```python
from build123d import *

# Parameters (mm, degrees)
SKETCH1_R                               = 159
SKETCH1_R_2                             = 121
BOSS_EXTRUDE1_DEPTH                     = 10
CBORE_FOR_M5_HEX_HEAD_BOLT2_D           = 6
CBORE_FOR_M5_HEX_HEAD_BOLT2_DEPTH       = 13
CBORE_FOR_M5_HEX_HEAD_BOLT2_CBORE_D     = 12
CBORE_FOR_M5_HEX_HEAD_BOLT2_CBORE_DEPTH = 6
CBORE_FOR_M5_HEX_HEAD_BOLT2_TIP         = 1.802581857


with BuildPart() as part:
    # Sketch1 → Boss-Extrude1 (new body)
    with BuildSketch(Plane(origin=(0, 0, 0), x_dir=(0, 0, -1), z_dir=(1, 0, 0))):
        Circle(SKETCH1_R)
        Circle(SKETCH1_R_2, mode=Mode.SUBTRACT)
    extrude(amount=BOSS_EXTRUDE1_DEPTH)

    # CBORE for M5 Hex Head Bolt2
    with Locations(Plane.ZY):
        with Locations((0, 150), (129.903810568, 75), (129.903810568, -75), (0, -150), (-129.903810568, -75), (-129.903810568, 75), (0, 0)):
            CounterBoreHole(CBORE_FOR_M5_HEX_HEAD_BOLT2_D / 2, CBORE_FOR_M5_HEX_HEAD_BOLT2_CBORE_D / 2, CBORE_FOR_M5_HEX_HEAD_BOLT2_CBORE_DEPTH, depth=CBORE_FOR_M5_HEX_HEAD_BOLT2_DEPTH)
            with Locations((0, 0, -(CBORE_FOR_M5_HEX_HEAD_BOLT2_DEPTH + CBORE_FOR_M5_HEX_HEAD_BOLT2_TIP / 2))):  # 118° drill point
                Cone(0, CBORE_FOR_M5_HEX_HEAD_BOLT2_D / 2, CBORE_FOR_M5_HEX_HEAD_BOLT2_TIP, mode=Mode.SUBTRACT)


solid = part.part
```
Design review of the part built by this model. Coordinates are the model's own, in mm. A direction names the side the tool comes from. Give positions to 0.01 mm unless a question says otherwise; leave off trailing zeros. Loops run counter-clockwise (first coordinate to the right, second up) from the corner with the lowest first, then second, coordinate; pieces in that order, holes last. Notation, with made-up numbers: (55.25, -21) -> (112.25, -21) arc R28 cw to (112.25, 2) -> close; hole circle Ø11 at (71, -1.5). An arc over 180 degrees is marked (long way). Write each question's results on one line, items separated by ' | '.
Q1. Machinability: for faces 4 (the face through (4.93, -118.123, 26.23)), 5 (the face through (6, -76, -133)), which of the approach directions +Z, -Z, +X, -X, +Y, -Y give a long, thin tool a straight path to every point of the face, cutting with its end or side? Answer none if there is none.
Reply:
face 4: +X, -X | face 5: -X
Q2. Take a section at A-A, the plane y = 0. Write out the cut boundary in (x, z), plus the area to 3 significant figures.
Reply:
outline: (0, -159) -> (10, -159) -> (10, -121) -> (0, -121) -> close; (0, 121) -> (10, 121) -> (10, 159) -> (0, 159) -> close | area: 760 mm²
Q3. Wall thickness on L1, parallel to Y at x = 4.05, z = 0; L2, parallel to Y at x = 1.25, z = 128.5; L3, parallel to Z at x = 9.75, y = -76: over which ranges is each line inside the solid? List them lowest first.
Reply:
L1: y = -159 to -156, -144 to -121, 121 to 144, 156 to 159 | L2: y = -93.64 to -80.83, -69.17 to 69.17, 80.83 to 93.64 | L3: z = -139.66 to -132.73, -127.08 to -94.15, 94.15 to 127.08, 132.73 to 139.66
Q4. For pin 1 Ø19 at (y, z) = (-75, 129.9) entering from +X; pin 2 Ø3 at (x, y) = (7.5, -19.5) entering from -Z; pin 3 Ø11 at (y, z) = (-150, 0) entering from -X; pin 4 Ø5 at (x, y) = (3, 23.5) entering from -Z, all flat-tipped, find the tip position at first contact; note any pin that passes through.
Reply:
pin 1: stops at x = 10 | pin 2: stops at z = -157.98 | pin 3: stops at x = 6 | pin 4: stops at z = -157.61
Q5. Take a section at B-B, the plane x = 7.5. Write out the cut boundary in (y, z).
Reply:
outline: circle Ø318 at (0, 0); hole circle Ø6 at (-150, 0); hole circle Ø242 at (0, 0); hole circle Ø6 at (-75, -129.9); hole circle Ø6 at (-75, 129.9); hole circle Ø6 at (75, -129.9); hole circle Ø6 at (75, 129.9); hole circle Ø6 at (150, 0)
Q6. The part is to be moulded in two halves that separate along Z. For faces 1 (the face through (0, -117, -35)), 2 (the face through (4.93, 157.647, 20.699)), 3 (the face through (6, -147, 1)), say which applies: +Z half, -Z half, draft (parallel to the pull), parting line (faces both ways), or undercut.
Reply:
face 1: draft | face 2: parting line | face 3: undercut
Q7. Take a section at C-C, the plane z = -89. Write out the cut boundary in (x, y), plus the area to 3 significant figures.
Reply:
outline: (0, -131.76) -> (10, -131.76) -> (10, -81.98) -> (0, -81.98) -> close; (0, 81.98) -> (10, 81.98) -> (10, 131.76) -> (0, 131.76) -> close | area: 996 mm²
